Build history of the part. All positions in model axes, mm. Coordinates: 2 decimals unless noted, no trailing zeros. Loops run counter-clockwise (first coordinate to the right, second up) from the corner with the lowest first, then second, coordinate; pieces in that order, holes last.
Item 1: Cut at B-B (x = 120). List the corners of the cut face in (y, z), and give its area (3 significant figures).
Item 2: Cut at D-D (y = 1.5). List the corners of the cut face in (x, z), and give its area (3 significant figures).
Item 3: Flat gauge pins, fed straight in: pin 1 (8 mm diameter, centred on x = 120, z = -40, fed in from +Y); pin 2 (16 mm diameter, centred on x = 40, z = -40, fed in from +Y). Where does each tip first touch, or does it go through?
Item 4: Mould opens along Z. For faces 1 (the face through (-60, 4, 1)), 2 (the face through (39, 4, -60)), 3 (the face through (-45, 4, 40)) say: released by +Z, released by -Z, zero draft, split by the parting line, or undercut.
Item 5: Cut at A-A (z = -40). List the corners of the cut face in (x, y), and give its area (3 significant figures).
Item 6: Drill centre lines: line 1 along X through (y, z) = (5.5, -40); line 2 along Z through (x, y) = (40, 5.5); line 3 along X through (y, z) = (4.75, 38.5). Where is each one in solid material? Low to high.
Item 7: Cut at C-C (x = 0). List the corners of the cut face in (y, z), and give its area (3 significant figures).
from build123d import *

# Parameters (mm, degrees)
SKETCH2_W            = 200
SKETCH2_H            = 120
BOSS_EXTRUDE3_DEPTH  = 8
SKETCH3_R            = 5
CUT_EXTRUDE1_DEPTH   = 9
LPATTERN2_COUNT      = 2
LPATTERN2_PITCH      = 80
LPATTERN2_COUNT_DIR2 = 3
LPATTERN2_PITCH_DIR2 = 80
SKETCH4_R            = 12.5
CUT_EXTRUDE2_DEPTH   = 10


with BuildPart() as part:
    # Sketch2 → Boss-Extrude3 (new body)
    with BuildSketch(Plane(origin=(0, 0, 0), x_dir=(1, 0, 0), z_dir=(0, 1, 0))):
        with Locations((40, 0)):
            Rectangle(SKETCH2_W, SKETCH2_H)
    extrude(amount=BOSS_EXTRUDE3_DEPTH)

    # Sketch3 → Cut-Extrude1 (cut, through all)
    with BuildSketch(Plane(origin=(0, 8, 0), x_dir=(1, 0, 0), z_dir=(0, 1, 0))):
        with Locations((-40, 40)):
            Circle(SKETCH3_R)
    cut_extrude1 = extrude(amount=-CUT_EXTRUDE1_DEPTH, mode=Mode.SUBTRACT)

    # LPattern2: Cut-Extrude1 2 × 3
    with Locations(*[(j * LPATTERN2_PITCH_DIR2, 0, i * LPATTERN2_PITCH) for i in range(LPATTERN2_COUNT) for j in range(LPATTERN2_COUNT_DIR2) if (i, j) != (0, 0)]):
        add(cut_extrude1, mode=Mode.SUBTRACT)

    # Sketch4 → Cut-Extrude2 (cut)
    with BuildSketch(Plane(origin=(0, 8, 0), x_dir=(1, 0, 0), z_dir=(0, 1, 0))):
        Circle(SKETCH4_R)
    extrude(amount=-CUT_EXTRUDE2_DEPTH, mode=Mode.SUBTRACT)


solid = part.part
Filled sheet:
1. outline: (0, -60) - (8, -60) - (8, -45) - (0, -45) - close; (0, -35) - (8, -35) - (8, 35) - (0, 35) - close; (0, 45) - (8, 45) - (8, 60) - (0, 60) - close
1. area: 800 mm2
2. outline: (-60, -60) - (140, -60) - (140, 60) - (-60, 60) - close; hole circle Ø10 at (-40, -40); hole circle Ø10 at (-40, 40); hole circle Ø25 at (0, 0); hole circle Ø10 at (40, -40); hole circle Ø10 at (40, 40); hole circle Ø10 at (120, -40); hole circle Ø10 at (120, 40)
2. area: 23,000 mm2
3. pin 1: passes through
3. pin 2: stops at y = 8
4. face 1: zero draft
4. face 2: released by -Z
4. face 3: undercut
5. outline: (-60, 0) - (-45, 0) - (-45, 8) - (-60, 8) - close; (-35, 0) - (35, 0) - (35, 8) - (-35, 8) - close; (45, 0) - (115, 0) - (115, 8) - (45, 8) - close; (125, 0) - (140, 0) - (140, 8) - (125, 8) - close
5. area: 1,360 mm2
6. line 1: x = -60 to -45, -35 to 35, 45 to 115, 125 to 140
6. line 2: z = -60 to -45, -35 to 35, 45 to 60
6. line 3: x = -60 to -44.77, -35.23 to 35.23, 44.77 to 115.23, 124.77 to 140
7. outline: (0, -60) - (8, -60) - (8, -12.5) - (0, -12.5) - close; (0, 12.5) - (8, 12.5) - (8, 60) - (0, 60) - close
7. area: 760 mm2
